```python
from build123d import *

# Parameters (mm, degrees)
CROQUIS1_R              = 3
CROQUIS1_R_2            = 2.5
SALIENTE_EXTRUIR1_DEPTH = 10
CROQUIS2_W              = 4.622971646
CROQUIS2_H              = 50
SALIENTE_EXTRUIR2_DEPTH = 5


with BuildPart() as part:
    # Croquis1 → Saliente-Extruir1 (new body)
    with BuildSketch(Plane.XY):
        Circle(CROQUIS1_R)
        Circle(CROQUIS1_R_2, mode=Mode.SUBTRACT)
    extrude(amount=SALIENTE_EXTRUIR1_DEPTH)

    # Croquis2 → Saliente-Extruir2 (add)
    with BuildSketch(Plane.XY.offset(10)):
        with Locations((-0.002035099, 23.090125411)):
            Rectangle(CROQUIS2_W, CROQUIS2_H)
    extrude(amount=SALIENTE_EXTRUIR2_DEPTH)


solid = part.part
```
Source: CAD feature listing. Evaluate the final solid. Frame: model axes, mm. A direction names the side the tool comes from. Coordinates: 2 decimals unless noted, no trailing zeros. Write each loop counter-clockwise with the first axis right and the second up, starting at its lowest first coordinate (ties: lowest second). Pieces come first, ordered by that corner, then holes. Notation, with made-up numbers: (74.25, -4) -> (123.25, -4) arc R34 cw to (123.25, 27) -> close; hole circle Ø3 at (26.5, 0). An arc over 180 degrees is marked (long way). Return JSON: item names as keys, results as strings. Group by question number.
1) Section query B-B, the plane x = 0. Return loops of the section in (y, z).
2) Section query D-D, the plane z = 12. Return loops of the section in (x, y), plus the area to 3 significant figures.
3) Section query C-C, the plane z = 4.5. Return loops of the section in (x, y), plus the area to 3 significant figures.
4) Section query A-A, the plane y = 0. Return loops of the section in (x, z), plus the area to 3 significant figures.
5) Set-up query: faces 5 (the face through (1.5, -2.2, 10)), 6 (the face through (-0.54, -2.44, 4.93)), 7 (the face through (0, -1.91, 12)). Return all of +Z, -Z, +X, -X, +Y, -Y with unobstructed straight access to the full face (end or side cutting, diameter ignored); none if empty.
6) Ray query, line 1 along Y through (x, z) = (0, 5.5); line 2 along Z through (x, y) = (-0.7, 26). Return the intervals inside material, ascending.
7) Contact query for flat-ended pins moving along their axis: P1, Ø1.4, axis at x = -0.5, y = 34, coming from the -Z side; P2, Ø5.5, axis at y = 29, z = 13, coming from the -X side; P3, Ø5.5, axis at y = 26, z = 12, coming from the +X side. Output: stop coordinate, or through.
8) Mould query, pull axis X, two halves, no side actions, for faces 1 (the face through (-3, 0, 5)), 2 (the face through (-2.314, 23, 12)), 3 (the face through (0, 23, 15)), 4 (the face through (0, 0, 10)). Classes: +X half, -X half, draft (parallel to the pull), parting line (faces both ways), or undercut.
From the geometry:
{
 "1": {"outline": "(-3, 0) -> (-2.5, 0) -> (-2.5, 10) -> (-3, 10) -> close; (-1.91, 10) -> (2.5, 10) -> (2.5, 0) -> (3, 0) -> (3, 10) -> (48.09, 10) -> (48.09, 15) -> (-1.91, 15) -> close"},
 "2": {"outline": "(-2.31, -1.91) -> (2.31, -1.91) -> (2.31, 48.09) -> (-2.31, 48.09) -> close", "area": "231 mm²"},
 "3": {"outline": "circle Ø6 at (0, 0); hole circle Ø5 at (0, 0)", "area": "8.64 mm²"},
 "4": {"outline": "(-3, 0) -> (-2.5, 0) -> (-2.5, 10) -> (-3, 10) -> close; (-2.31, 10) -> (2.31, 10) -> (2.31, 15) -> (-2.31, 15) -> close; (2.5, 0) -> (3, 0) -> (3, 10) -> (2.5, 10) -> close", "area": "33.1 mm²"},
 "5": {"face 5": "+Z, +X, -Y", "face 6": "-Z", "face 7": "+Z, +X, -X, -Y"},
 "6": {"line 1": "-3 to -2.5, 2.5 to 3", "line 2": "10 to 15"},
 "7": {"P1": "z = 10", "P2": "x = -2.31", "P3": "x = 2.31"},
 "8": {"face 1": "parting line", "face 2": "-X half", "face 3": "draft", "face 4": "undercut"}
}
